from build123d import *

# Parameters (mm, degrees)
F0_R      = 136.5
F0_R_2    = 131.5
F1_DEPTH  = 600
F3_R      = 131.5
F4_DEPTH  = 8
F5_R      = 25
F6_DEPTH  = 400
F7_R      = 15
F8_DEPTH  = 154
F9_DEPTH  = 149
F10_R     = 125
F11_DEPTH = 348
F12_R     = 175
F12_R_2   = 136.5
F13_DEPTH = 1133
F15_R     = 136.5
F15_R_2   = 25
F16_DEPTH = 8


with BuildPart() as f1:
    # F0 (on Front) → F1 (new body)
    with BuildSketch(Plane.XZ):
        Circle(F0_R)
        Circle(F0_R_2, mode=Mode.SUBTRACT)
    extrude(amount=F1_DEPTH)

    # F3 (on offset) → F4 (join)
    with BuildSketch(Plane.XZ.offset(500)):
        Circle(F3_R)
    extrude(amount=F4_DEPTH)

    # F5 (on face) → F6 (join)
    with BuildSketch(Plane.XZ.offset(508)):
        Circle(F5_R)
    extrude(amount=F6_DEPTH)

    # F7 (on Right) → F8 (join)
    with BuildSketch(Plane.YZ):
        with Locations((-310, 0)):
            Circle(F7_R)
    extrude(amount=F8_DEPTH)

    # F7 (on Right) → F9 (join)
    with BuildSketch(Plane.YZ):
        with Locations((-310, 0)):
            Circle(F7_R)
    extrude(amount=-F9_DEPTH)

    # F10 (on face) → F11 (cut)
    with BuildSketch(Plane.YZ.offset(154)):
        with Locations((-310, 150)):
            Circle(F10_R)
    extrude(amount=-F11_DEPTH, mode=Mode.SUBTRACT)

    # F12 (on face) → F13 (cut)
    with BuildSketch(Plane.XZ.offset(908)):
        Circle(F12_R)
        Circle(F12_R_2, mode=Mode.SUBTRACT)
    extrude(amount=-F13_DEPTH, mode=Mode.SUBTRACT)

    # F15 (on offset) → F16 (join)
    with BuildSketch(Plane.XZ.offset(590)):
        Circle(F15_R)
        Circle(F15_R_2, mode=Mode.SUBTRACT)
    extrude(amount=-F16_DEPTH)


solid = f1.part
Read the model definition and answer for the solid it produces. Units are mm, in the model's axes. A direction names the side the tool comes from. Coordinates: 2 decimals unless noted, no trailing zeros. Write each loop counter-clockwise with the first axis right and the second up, starting at its lowest first coordinate (ties: lowest second). Pieces come first, ordered by that corner, then holes. Notation, with made-up numbers: (56.25, 3.25) - (80.25, 3.25) arc R17 ccw to (80.25, 13.25) - close; hole circle Ø11 at (65.5, -16). An arc over 180 degrees is marked (long way). One line per question, with ' | ' between items.
Q1. Find section B-B, the plane y = -553. Write down the section's boundary in (x, z).
Result set:
outline: circle Ø273 at (0, 0); circle Ø50 at (0, 0); hole circle Ø263 at (0, 0)
Q2. Each of these flat-tipped pins is pushed along its axis until it touches: P1, Ø6, axis at x = -6.5, y = -372.5, coming from the +Z side; P2, Ø10, axis at x = -27.5, y = -567.5, coming from the -Z side; P3, Ø6, axis at x = 58.5, y = -566.5, coming from the +Z side. Where does it stop, or does it pass through?
Result set:
P1: z = -131.16 | P2: z = -134.63 | P3: z = 124.71
Q3. Find section A-A, the plane x = 109. Write down the section's boundary in (y, z).
Result set:
outline: (-600, -82.17) - (0, -82.17) - (0, -73.56) - (-500, -73.56) - (-500, 73.56) - (-408.9, 73.56) arc R125 cw to (-414.99, 82.17) - (-600, 82.17) - (-600, 73.56) - (-590, 73.56) - (-590, -73.56) - (-600, -73.56) - close; circle Ø30 at (-310, 0); (-211.1, 73.56) - (0, 73.56) - (0, 82.17) - (-205.01, 82.17) arc R125 cw to start; hole (-582, -73.56) - (-508, -73.56) - (-508, 73.56) - (-582, 73.56) - close
Q4. Consider L1, parallel to Z at x = 0, y = -596; L2, parallel to Y at x = -4, z = 118; L3, parallel to Y at x = 54, z = 0.5. Determine where each line is inside the solid, lowest interval first. Write a range as [from, to].
Result set:
L1: [-136.5, -131.5], [-25, 25], [131.5, 136.5] | L2: [-590, -582], [-508, -500] | L3: [-590, -582], [-508, -500], [-324.99, -295.01]
Q5. Find section C-C, the plane x = 0. State how many separate pieces and enclosed holes the cut face has, plus the area to 3 significant figures.
Result set:
separate pieces: 3 | enclosed holes: 2 | area: 29,300 mm^2
Q6. Find section D-D, the plane z = 68.5. Write down the section's boundary in (x, y), plus the area to 3 significant figures.
Result set:
outline: (-118.07, -600) - (-112.25, -600) - (-112.25, -590) - (112.25, -590) - (112.25, -600) - (118.07, -600) - (118.07, -404.78) - (112.25, -404.78) - (112.25, -500) - (-112.25, -500) - (-112.25, -404.78) - (-118.07, -404.78) - close; (-118.07, -215.22) - (-112.25, -215.22) - (-112.25, 0) - (-118.07, 0) - close; (112.25, -215.22) - (118.07, -215.22) - (118.07, 0) - (112.25, 0) - close; hole (-112.25, -582) - (112.25, -582) - (112.25, -508) - (-112.25, -508) - close | area: 8,370 mm^2
Q7. Determine the mould class of faces 1 (the flat face through (-112, -600, 71)), 2 (the cylindrical face through (23.846, -746.774, 7.509)), 3 (the flat face through (27, -508, 2)) for opening direction Y: +Y half, -Y half, draft (parallel to the pull), parting line (faces both ways), or undercut.
Result set:
face 1: -Y half | face 2: draft | face 3: undercut
Q8. For faces 4 (the cylindrical face through (23.846, -544.482, 7.509)), 5 (the cylindrical face through (-29.591, -304.2, -133.254)), 6 (the cylindrical face through (70.694, -594.93, 110.881)), determine the directions among +Z, -Z, +X, -X, +Y, -Y from which every point of the face is accessible in a straight line to the end or side of a thin tool.
Result set:
face 4: none | face 5: +Y, -Y | face 6: -Y
